Can you work these out from the model? Positions are in its coordinate system, mm. A direction names the side the tool comes from. Round coordinates to 2 decimals unless told otherwise and drop trailing zeros. Loops run counter-clockwise (first coordinate to the right, second up) from the corner with the lowest first, then second, coordinate; pieces in that order, holes last. Notation, with made-up numbers: (80.25, -16.5) - (111.25, -16.5) arc R28 cw to (111.25, 3.5) - close; hole circle Ø3 at (79, -1.75). An arc over 180 degrees is marked (long way). Answer as CSV lines item,"result".
```python
from build123d import *

# Parameters (mm, degrees)
BOSS_EXTRU_1_DEPTH      = 60
ESQUISSE2_R             = 30
ESQUISSE2_R_2           = 29
BOSS_EXTRU_2_DEPTH      = 60
ESQUISSE3_R             = 25
ENL_V_MAT_EXTRU_1_DEPTH = 27
ESQUISSE6_R             = 2.225
ENL_V_MAT_EXTRU_3_DEPTH = 2
ESQUISSE10_W            = 42
ESQUISSE10_H            = 21.645898034
ENL_V_MAT_EXTRU_7_DEPTH = 5


with BuildPart() as part:
    # Esquisse1 → Boss.-Extru.1 (new body)
    with BuildSketch(Plane.XY):
        with BuildLine():
            Line((1, -15.006468588), (1, -3.354101966))
            ThreePointArc((1, -3.354101966), (3.5, 0), (1, 3.354101966))
            Line((1, 3.354101966), (1, 29.5))
            Line((1, 29.5), (-1, 29.5))
            Line((-1, 29.5), (-1, 3.354101966))
            ThreePointArc((-1, 3.354101966), (-3.5, 0), (-1, -3.354101966))
            Line((-1, -3.354101966), (-1, -29.5))
            Line((-1, -29.5), (1, -29.5))
            Line((1, -29.5), (1, -15.006468588))
        make_face()
    extrude(amount=BOSS_EXTRU_1_DEPTH)

    # Esquisse2 → Boss.-Extru.2 (add)
    with BuildSketch(Plane.XY.offset(60)):
        Circle(ESQUISSE2_R)
        Circle(ESQUISSE2_R_2, mode=Mode.SUBTRACT)
    extrude(amount=-BOSS_EXTRU_2_DEPTH)

    # Esquisse3 → Enlèv. mat.-Extru.1 (cut)
    with BuildSketch(Plane.XY.offset(60)):
        Circle(ESQUISSE3_R)
    extrude(amount=-ENL_V_MAT_EXTRU_1_DEPTH, mode=Mode.SUBTRACT)

    # Esquisse6 → Enlèv. mat.-Extru.3 (cut)
    with BuildSketch(Plane.XY.offset(33)):
        Circle(ESQUISSE6_R)
    extrude(amount=-ENL_V_MAT_EXTRU_3_DEPTH, mode=Mode.SUBTRACT)

    # Esquisse10 → Enlèv. mat.-Extru.7 (cut)
    with BuildSketch(Plane(origin=(1, 0, 0), x_dir=(0, 0, -1), z_dir=(1, 0, 0))):
        with Locations((-39, -14.177050983)):
            Rectangle(ESQUISSE10_W, ESQUISSE10_H)
        with Locations((-39, 14.177050983)):
            Rectangle(ESQUISSE10_W, ESQUISSE10_H)
    extrude(amount=-ENL_V_MAT_EXTRU_7_DEPTH, mode=Mode.SUBTRACT)


solid = part.part
```
Q1. Imagine slicing it at C-C (x = 0). Write out the boundary of the cut face in (y, z) (3 decimals), then the cut area to 3 significant figures.
Checks:
outline,"(-30, 0) - (30, 0) - (30, 60) - (25, 60) - (25, 18) - (3.354, 18) - (3.354, 33) - (2.225, 33) - (2.225, 31) - (-2.225, 31) - (-2.225, 33) - (-3.354, 33) - (-3.354, 18) - (-25, 18) - (-25, 60) - (-30, 60) - close"
area,"1,590 mm²"
Q2. We'd pull the mould along X, two halves only. Please class faces 4 (the flat face through (-2, 0, 0)), 5 (the flat face through (0, 0, 31)): pulls with the +X half, pulls with the -X half, needs draft (parallel to the pull), parting line crosses it, or undercut.
Checks:
face 4,"needs draft"
face 5,"undercut"
Q3. If I drill on line 1 along Y through (x, z) = (0, 32) (3 decimals); line 2 along X through (y, z) = (25.5, 35); line 3 along X through (y, z) = (12, 14.5), over which ranges is the centre line in solid material (lowest first)? Write a range as [from, to].
Checks:
line 1,"[-30, -25], [-3.354, -2.225], [2.225, 3.354], [25, 30]"
line 2,"[-15.8, -13.81], [-1, 1], [13.81, 15.8]"
line 3,"[-27.5, -26.4], [-1, 1], [26.4, 27.5]"
Q4. Imagine slicing it at D-D (x = 14). Write out the boundary of the cut face in (y, z), then the cut area to 3 significant figures.
Checks:
outline,"(-26.53, 0) - (-25.4, 0) - (-25.4, 60) - (-26.53, 60) - close; (25.4, 0) - (26.53, 0) - (26.53, 60) - (25.4, 60) - close"
area,"136 mm²"
Q5. On a 3-axis mill with a long thin cutter (end or side, diameter ignored), from which of +Z, -Z, +X, -X, +Y, -Y can I reach the whole of each face in a straight line? I mean faces 1 (the flat face through (0, -3.354, 26)), 2 (the flat face through (0, 27, 60)), 3 (the flat face through (1, -19, 16)). Say none if no direction works.
Checks:
face 1,"+Z"
face 2,"+Z, +X, -X, +Y, -Y"
face 3,"+Z, -Z"
Q6. I'm going to push flat-ended pins straight in: pin 1 Ø1.6 at (x, z) = (0, 23) entering from +Y; pin 2 Ø1.5 at (y, z) = (18, 50) entering from +X; pin 3 Ø7.5 at (y, z) = (-22, 41.5) entering from +X; pin 4 Ø12 at (x, y) = (24, -23.5) entering from +Z. Where does each tip first touch, or does it pass through?
Checks:
pin 1,"y = 30"
pin 2,"x = 24.54"
pin 3,"x = 23.81"
pin 4,"z = 60"
Q7. Imagine slicing it at A-A (y = 0). Write out the boundary of the cut face in (x, z) (3 decimals).
Checks:
outline,"(-30, 0) - (-29, 0) - (-29, 60) - (-30, 60) - close; (-3.5, 0) - (3.5, 0) - (3.5, 33) - (2.225, 33) - (2.225, 31) - (-2.225, 31) - (-2.225, 33) - (-3.5, 33) - close; (29, 0) - (30, 0) - (30, 60) - (29, 60) - close"
